For this review, take the finished solid that the model builds, in its own axes (mm). A direction names the side the tool comes from. Round coordinates to 2 decimals unless told otherwise and drop trailing zeros. Order: outer loops, then holes, each group sorted by start corner. A loop starts at its lowest first (then second) coordinate and runs counter-clockwise, first axis right, second up. Notation, with made-up numbers: M -32,59.25 L 9,59.25 A22 ccw 9,91.25 Z; hole C -7,-10.5 d6. An arc over 180 degrees is marked long. Answer in a Markdown table with one row per item. Add a question column.
```python
from build123d import *

# Parameters (mm, degrees)
SKETCH1_W           = 400
SKETCH1_H           = 70
BOSS_EXTRUDE1_DEPTH = 30
CUT_EXTRUDE1_DEPTH  = 20
FILLET1_R           = 0.1
FILLET2_START       = 10
FILLET2_DEPTH       = 21
BOSS_EXTRUDE2_DEPTH = 20
LPATTERN1_COUNT     = 4
LPATTERN1_PITCH     = 100
BOSS_EXTRUDE3_DEPTH = 20
LPATTERN2_COUNT     = 3
LPATTERN2_PITCH     = 100
SKETCH5_R           = 10
BOSS_EXTRUDE4_DEPTH = 20
SKETCH6_W           = 400
SKETCH6_H           = 70
BOSS_EXTRUDE5_DEPTH = 1


with BuildPart() as part:
    # Sketch1 → Boss-Extrude1 (new body)
    with BuildSketch(Plane.XY):
        Rectangle(SKETCH1_W, SKETCH1_H)
    extrude(amount=BOSS_EXTRUDE1_DEPTH)

    # Sketch2 → Cut-Extrude1 (cut)
    with BuildSketch(Plane.XY.offset(30)):
        with BuildLine():
            Line((-128.697541479, 4.604917042), (-175, -5))
            Line((-175, -5), (-200, -5))
            Line((-200, -5), (-200, 5))
            Line((-200, 5), (-190.811388301, 5))
            ThreePointArc((-190.811388301, 5), (-187.890958939, 24.335251481), (-168.875, 28.893119746))
            Line((-168.875, 28.893119746), (-81.125, -3.893119746))
            ThreePointArc((-81.125, -3.893119746), (-91.393119746, 18.625), (-68.875, 28.893119746))
            Line((-68.875, 28.893119746), (18.875, -3.893119746))
            ThreePointArc((18.875, -3.893119746), (8.606880254, 18.625), (31.125, 28.893119746))
            Line((31.125, 28.893119746), (118.875, -3.893119746))
            ThreePointArc((118.875, -3.893119746), (108.53578111, 18.431230593), (130.736636107, 29.033027738))
            Line((130.736636107, 29.033027738), (200, 5))
            Line((200, 5), (200, -5))
            Line((200, -5), (189.969387627, -21.564625424))
            ThreePointArc((189.969387627, -21.564625424), (161.524837834, -23.665572292), (168.875, 3.893119746))
            Line((168.875, 3.893119746), (81.125, -28.893119746))
            ThreePointArc((81.125, -28.893119746), (58.606880254, -18.625), (68.875, 3.893119746))
            Line((68.875, 3.893119746), (-18.875, -28.893119746))
            ThreePointArc((-18.875, -28.893119746), (-41.393119746, -18.625), (-31.125, 3.893119746))
            Line((-31.125, 3.893119746), (-118.875, -28.893119746))
            ThreePointArc((-118.875, -28.893119746), (-141.792937679, -17.424149076), (-128.697541479, 4.604917042))
        make_face()
    extrude(amount=-CUT_EXTRUDE1_DEPTH, mode=Mode.SUBTRACT)

    # Fillet1
    fillet1_edges = [part.edges().sort_by_distance(p)[0] for p in [
        (-128.697541479, 4.604917042, 20),
    ]]
    fillet(fillet1_edges, radius=FILLET1_R)

    # Fillet2: read off the stored shape, not the designer's step
    # Fillet2 outline → Fillet2 (cut)
    with BuildSketch(Plane.XY.offset(FILLET2_START)):
        with BuildLine():
            ThreePointArc((-33.603406746, 2.967106787), (-33.477636502, 2.91539326), (-33.519722617, 2.786082773))
            ThreePointArc((-33.519722617, 2.786082773), (-32.343252539, 3.384792796), (-31.125, 3.893119746))
            Line((-31.125, 3.893119746), (-33.603406746, 2.967106787))
        make_face()
        with BuildLine():
            ThreePointArc((66.396593254, 2.967106787), (66.522363498, 2.91539326), (66.480277383, 2.786082773))
            ThreePointArc((66.480277383, 2.786082773), (67.656747461, 3.384792796), (68.875, 3.893119746))
            Line((68.875, 3.893119746), (66.396593254, 2.967106787))
        make_face()
        with BuildLine():
            ThreePointArc((166.396593254, 2.967106787), (166.522363498, 2.91539326), (166.480277383, 2.786082773))
            ThreePointArc((166.480277383, 2.786082773), (167.656747461, 3.384792796), (168.875, 3.893119746))
            Line((168.875, 3.893119746), (166.396593254, 2.967106787))
        make_face()
        with BuildLine():
            ThreePointArc((116.480277383, -2.786082773), (116.522363498, -2.91539326), (116.396593254, -2.967106787))
            Line((116.396593254, -2.967106787), (118.875, -3.893119746))
            ThreePointArc((118.875, -3.893119746), (117.656747461, -3.384792796), (116.480277383, -2.786082773))
        make_face()
        with BuildLine():
            ThreePointArc((-81.125, -3.893119746), (-82.343252539, -3.384792796), (-83.519722617, -2.786082773))
            ThreePointArc((-83.519722617, -2.786082773), (-83.477636502, -2.91539326), (-83.603406746, -2.967106787))
            Line((-83.603406746, -2.967106787), (-81.125, -3.893119746))
        make_face()
        with BuildLine():
            ThreePointArc((16.480277383, -2.786082773), (16.522363498, -2.91539326), (16.396593254, -2.967106787))
            Line((16.396593254, -2.967106787), (18.875, -3.893119746))
            ThreePointArc((18.875, -3.893119746), (17.656747461, -3.384792796), (16.480277383, -2.786082773))
        make_face()
    extrude(amount=FILLET2_DEPTH, mode=Mode.SUBTRACT)

    # Sketch3 → Boss-Extrude2 (add)
    with BuildSketch(Plane.XY.offset(10)):
        with BuildLine():
            Line((-171, 3.33484861), (-150, 12.5))
            Line((-150, 12.5), (-171, 21.66515139))
            ThreePointArc((-171, 21.66515139), (-185, 12.5), (-171, 3.33484861))
        make_face()
    boss_extrude2 = extrude(amount=BOSS_EXTRUDE2_DEPTH)

    # LPattern1: Boss-Extrude2 ×4
    with Locations(*[(i * LPATTERN1_PITCH, 0, 0) for i in range(1, LPATTERN1_COUNT)]):
        add(boss_extrude2)

    # Sketch4 → Boss-Extrude3 (add)
    with BuildSketch(Plane.XY.offset(10)):
        with BuildLine():
            Line((-121, -21.66515139), (-100, -12.5))
            Line((-100, -12.5), (-121, -3.33484861))
            ThreePointArc((-121, -3.33484861), (-135, -12.5), (-121, -21.66515139))
        make_face()
    boss_extrude3 = extrude(amount=BOSS_EXTRUDE3_DEPTH)

    # LPattern2: Boss-Extrude3 ×3
    with Locations(*[(i * LPATTERN2_PITCH, 0, 0) for i in range(1, LPATTERN2_COUNT)]):
        add(boss_extrude3)

    # Sketch5 → Boss-Extrude4 (add)
    with BuildSketch(Plane.XY.offset(10)):
        with Locations((175, -12.5)):
            Circle(SKETCH5_R)
    extrude(amount=BOSS_EXTRUDE4_DEPTH)

    # Sketch6 → Boss-Extrude5 (add)
    with BuildSketch(Plane.XY.offset(30)):
        Rectangle(SKETCH6_W, SKETCH6_H)
    extrude(amount=BOSS_EXTRUDE5_DEPTH)


solid = part.part
```
1. Consider section C-C on x = 175. Write out the cut boundary in (y, z), plus the area to 3 significant figures.
2. To check wall thickness, follow probe 1 along Z at (x, y) = (-176.5, -2.5); probe 2 along Y at (x, z) = (175, 20); probe 3 along Y at (x, z) = (-39.5, 28). State the ranges of each line that lie inside material, in increasing order. Write a range as [from, to].
3. Consider section A-A on x = 125. Write out the cut boundary in (y, z).
4. The part is to be moulded in two halves that separate along Z. For faces 1 (the flat face through (-3, 0, 30)), 2 (the flat face through (-3, 0, 31)), 3 (the flat face through (200, 0, 8)), say which applies: pulls with the +Z half, pulls with the -Z half, needs draft (parallel to the pull), parting line crosses it, or undercut.
5. Consider section B-B on z = 23. State how many separate pieces and enclosed holes the cut face has, plus the area to 3 significant figures.
6. For faces 4 (the flat face through (-195, 5, 20)), 5 (the flat face through (139.35, 7.85, 19.86)), 6 (the flat face through (-200, 0, 8)), list the 3-axis set-ups (+Z, -Z, +X, -X, +Y, -Y) from which the entire face can be reached by the end or side of a thin tool; tool diameter is ignored.
Solved:
| question | item | result |
|---|---|---|
| 1 | outline | M -35,0 L 35,0 L 35,31 L -35,31 Z; hole M -30,10 L -22.5,10 L -22.5,30 L -30,30 Z; hole M -2.5,10 L 13.67,10 L 13.67,30 L -2.5,30 Z |
| 1 | area | 1,700 mm^2 |
| 2 | probe 1 | z = [0, 10], [30, 31] |
| 2 | probe 2 | y = [-35, -30], [-22.5, -2.5], [13.67, 35] |
| 2 | probe 3 | y = [-35, -22.3], [-2.7, 0.76], [17.92, 35] |
| 3 | outline | M -35,0 L 35,0 L 35,31 L -35,31 Z; hole M -12.5,10 L 2.5,10 L 2.5,30 L -12.5,30 Z; hole M 22.5,10 L 30,10 L 30,30 L 22.5,30 Z |
| 4 | face 1 | undercut |
| 4 | face 2 | pulls with the +Z half |
| 4 | face 3 | needs draft |
| 5 | separate pieces | 10 |
| 5 | enclosed holes | 0 |
| 5 | area | 17,900 mm^2 |
| 6 | face 4 | -X |
| 6 | face 5 | none |
| 6 | face 6 | +Z, -Z, -X, +Y, -Y |
